from build123d import *

# Parameters (mm, degrees)
BOSS_EXTRUDE1_DEPTH = 6
SKETCH2_W           = 55
SKETCH2_H           = 50
CUT_EXTRUDE1_DEPTH  = 10


with BuildPart() as part:
    # Sketch1 → Boss-Extrude1 (new body)
    with BuildSketch(Plane.XY):
        Polygon((28.571428571, 236.060202245), (28.571428571, 237.05184048), (5.415486436, 237.05184048), (4.571428571, 268.104761905), (-12.428571429, 268.104761905), (-12.428571429, 237.05184048), (-38.216595912, 237.05184048), (-38.216595912, 268.104761905), (-171.428571429, 268.104761905), (-171.428571429, 241.104761905), (-370.123537574, 241.104761905), (-370.123537574, -22.895238095), (28.571428571, -22.895238095), align=None)
    extrude(amount=BOSS_EXTRUDE1_DEPTH)

    # Sketch2 → Cut-Extrude1 (cut)
    with BuildSketch(Plane.XY.offset(6)):
        with Locations((-342.623537574, 216.104761905)):
            Rectangle(SKETCH2_W, SKETCH2_H)
    extrude(amount=-CUT_EXTRUDE1_DEPTH, mode=Mode.SUBTRACT)


solid = part.part
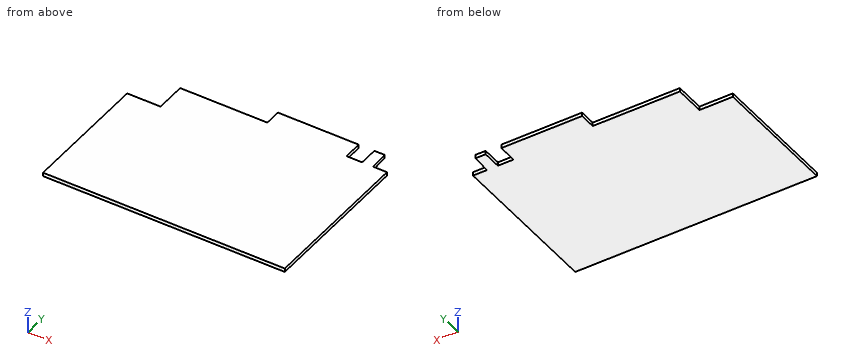
The model under review builds one solid part; all positions refer to its coordinate system, in mm. Give positions to 0.01 mm unless a question says otherwise; leave off trailing zeros. Write each loop counter-clockwise with the first axis right and the second up, starting at its lowest first coordinate (ties: lowest second). Pieces come first, ordered by that corner, then holes.
1. Add section B-B, the plane x = -255. Write out the cut boundary in (y, z), plus the area to 3 significant figures.
2. Add section A-A, the plane z = 1.75. Write out the cut boundary in (x, y), plus the area to 3 significant figures.
3. Wall thickness on L1, parallel to Y at x = -322, z = 3.75; L2, parallel to X at y = 212, z = 2.5; L3, parallel to Y at x = -289.5, z = 3.65: over which ranges is each line inside the solid? List them lowest first.
4. Add section C-C, the plane y = 217.5. Write out the cut boundary in (x, z), plus the area to 3 significant figures.
5. For P1, Ø3, axis at y = 247.5, z = 3, coming from the -X side; P2, Ø3, axis at x = -254.5, z = 4, coming from the +Y side, all flat-tipped, find the tip position at first contact; note any pin that passes through.
Worked answers:
1. outline: (-22.9, 0) - (241.1, 0) - (241.1, 6) - (-22.9, 6) - close
1. area: 1,580 mm2
2. outline: (-370.12, -22.9) - (28.57, -22.9) - (28.57, 237.05) - (5.42, 237.05) - (4.57, 268.1) - (-12.43, 268.1) - (-12.43, 237.05) - (-38.22, 237.05) - (-38.22, 268.1) - (-171.43, 268.1) - (-171.43, 241.1) - (-315.12, 241.1) - (-315.12, 191.1) - (-370.12, 191.1) - close
2. area: 106,000 mm2
3. L1: y = -22.9 to 191.1
3. L2: x = -315.12 to 28.57
3. L3: y = -22.9 to 241.1
4. outline: (-315.12, 0) - (28.57, 0) - (28.57, 6) - (-315.12, 6) - close
4. area: 2,060 mm2
5. P1: stops at x = -171.43
5. P2: stops at y = 241.1
